```python
from build123d import *

# Parameters (mm, degrees)
F0_W     = 106.7152023315
F0_H     = 67.4116164446
F1_DEPTH = 2
F2_D     = 5.5
F2_DEPTH = 18
F2_TIP   = 1.6523667023
F4_D     = 3.3
F4_DEPTH = 18
F4_TIP   = 0.9914200214


with BuildPart() as f1:
    # F0 (on Top) → F1 (new body)
    with BuildSketch(Plane.XY):
        with Locations((-19.7555795312, 1.5103928745)):
            Rectangle(F0_W, F0_H)
    extrude(amount=F1_DEPTH)

    # F2
    with Locations(Plane(origin=(0, 0, 0), x_dir=(1, 0, 0), z_dir=(0, 0, -1))):
        with Locations((-64.3030628562, -16.9964022934), (25.6969371438, -28.9964022934), (25.6969371438, 28.0035977066)):
            Hole(F2_D / 2, depth=F2_DEPTH)
            with Locations((0, 0, -(F2_DEPTH + F2_TIP / 2))):  # 118° drill point
                Cone(0, F2_D / 2, F2_TIP, mode=Mode.SUBTRACT)

    # F4
    with Locations(Plane.XY.offset(2)):
        with Locations((-56.4374391407, 27.3174114525), (17.1625608593, 27.3174114525), (-57.7374391407, -22.6825885475), (26.2625608593, -22.6825885475)):
            Hole(F4_D / 2, depth=F4_DEPTH)
            with Locations((0, 0, -(F4_DEPTH + F4_TIP / 2))):  # 118° drill point
                Cone(0, F4_D / 2, F4_TIP, mode=Mode.SUBTRACT)


solid = f1.part
```
Geometry check sheet. Reference: the model listing, model coordinates, mm. Coordinates: 2 decimals unless noted, no trailing zeros. Order: outer loops, then holes, each group sorted by start corner. A loop starts at its lowest first (then second) coordinate and runs counter-clockwise, first axis right, second up.
Item 1: Scan lines: line 1 along X through (y, z) = (-23, 1.45); line 2 along X through (y, z) = (-22, 1.55); line 3 along X through (y, z) = (19, 0.4). Record each from-to range of solid material in increasing order.
Item 2: Depth check by flat-ended pin: pin 1 (7 mm diameter, centred on x = 25.7, y = -28, fed in from +Z). Enter the tip coordinate at first touch or a pass-through.
Item 3: Mould release check, pull along X, two halves, no side actions. Record for faces 1 (the cylindrical face through (-62.276, 15.138, 1.014)), 2 (the flat face through (-21, 2, 0)), 3 (the flat face through (33.602, 1, 1)): released by +X, released by -X, zero draft, split by the parting line, or undercut.
Item 4: Section check A-A (y = 15.5). Enter the section's corners in (x, z).
Check sheet entries:
1. line 1: x = -73.11 to -59.36, -56.12 to 24.64, 27.88 to 33.6
1. line 2: x = -73.11 to -59.24, -56.24 to 24.76, 27.76 to 33.6
1. line 3: x = -73.11 to -66.19, -62.42 to 33.6
2. pin 1: stops at z = 2
3. face 1: undercut
3. face 2: zero draft
3. face 3: released by +X
4. outline: (-73.11, 0) - (-66.61, 0) - (-66.61, 2) - (-73.11, 2) - close; (-62, 0) - (33.6, 0) - (33.6, 2) - (-62, 2) - close
